from build123d import *

# Parameters (mm, degrees)
F2_DEPTH      = 24.25
F2_DEPTH_BACK = 24.25
F3_R          = 11.025
F3_R_2        = 1.75
F4_DEPTH      = 4.75
F6_DEPTH      = 15
F6_DEPTH_BACK = 15


with BuildPart() as f2:
    # F1 (on Front) → F2 (new body, two sides)
    with BuildSketch(Plane.XZ) as f2_sk:
        with BuildLine():
            ThreePointArc((-31.323529, -7.382294), (-30, 7.5), (-28.676471, -7.382294))
            ThreePointArc((-28.676471, -7.382294), (-29.266965, -7.724911), (-29.5, -8.3666))
            Line((-29.5, -8.3666), (-29.5, -11.401754))
            ThreePointArc((-29.5, -11.401754), (-29.15938, -12.153564), (-28.369565, -12.393211))
            ThreePointArc((-28.369565, -12.393211), (-19.18639, -6.270235), (-18.434131, 4.741379))
            ThreePointArc((-18.434131, 4.741379), (-18.244502, 6.614172), (-16.583592, 7.5))
            Line((-16.583592, 7.5), (16.583592, 7.5))
            ThreePointArc((16.583592, 7.5), (18.244502, 6.614172), (18.434131, 4.741379))
            ThreePointArc((18.434131, 4.741379), (19.18639, -6.270235), (28.369565, -12.393211))
            ThreePointArc((28.369565, -12.393211), (29.15938, -12.153564), (29.5, -11.401754))
            Line((29.5, -11.401754), (29.5, -8.3666))
            ThreePointArc((29.5, -8.3666), (29.266965, -7.724911), (28.676471, -7.382294))
            ThreePointArc((28.676471, -7.382294), (30, 7.5), (31.323529, -7.382294))
            ThreePointArc((31.323529, -7.382294), (30.733035, -7.724911), (30.5, -8.3666))
            Line((30.5, -8.3666), (30.5, -11.401754))
            ThreePointArc((30.5, -11.401754), (30.84062, -12.153564), (31.630435, -12.393211))
            ThreePointArc((31.630435, -12.393211), (40.81361, -6.270235), (41.565869, 4.741379))
            ThreePointArc((41.565869, 4.741379), (41.755498, 6.614172), (43.416408, 7.5))
            Line((43.416408, 7.5), (50, 7.5))
            Line((50, 7.5), (50, 12.5))
            Line((50, 12.5), (24.75, 12.5))
            Line((24.75, 12.5), (24.75, 82.5))
            Line((24.75, 82.5), (20, 82.5))
            Line((20, 82.5), (20, 12.5))
            Line((20, 12.5), (-43.416408, 12.5))
            Line((-43.416408, 12.5), (-43.416408, 7.5))
            ThreePointArc((-43.416408, 7.5), (-41.755498, 6.614172), (-41.565869, 4.741379))
            ThreePointArc((-41.565869, 4.741379), (-40.81361, -6.270235), (-31.630435, -12.393211))
            ThreePointArc((-31.630435, -12.393211), (-30.84062, -12.153564), (-30.5, -11.401754))
            Line((-30.5, -11.401754), (-30.5, -8.3666))
            ThreePointArc((-30.5, -8.3666), (-30.733035, -7.724911), (-31.323529, -7.382294))
        make_face()
    extrude(amount=F2_DEPTH)
    extrude(f2_sk.sketch, amount=-F2_DEPTH_BACK)

    # F3 (on face) → F4 (cut, through all)
    with BuildSketch(Plane(origin=(20, 0, 0), x_dir=(0, -1, 0), z_dir=(-1, 0, 0))):
        with Locations((1.9, 58.65)):
            Circle(F3_R)
        with Locations((-13.6, 43.15)):
            Circle(F3_R_2)
        with Locations((17.4, 43.15)):
            Circle(F3_R_2)
        with Locations((17.4, 74.15)):
            Circle(F3_R_2)
        with Locations((-13.6, 74.15)):
            Circle(F3_R_2)
    extrude(amount=-F4_DEPTH, mode=Mode.SUBTRACT)

    # F5 (on Front) → F6 (join, two sides)
    with BuildSketch(Plane.XZ) as f6_sk:
        Polygon((-10, -11.5), (-10, 9.493519), (-19.701663, 9.493519), (-19.701663, 0), (-27.352255, -11.5), align=None)
    extrude(amount=F6_DEPTH)
    extrude(f6_sk.sketch, amount=-F6_DEPTH_BACK)


solid = f2.part
Here's how the part is built. I have some questions about the finished solid (model axes, mm). A direction names the side the tool comes from. Give positions to 0.01 mm unless a question says otherwise; leave off trailing zeros. Loops run counter-clockwise (first coordinate to the right, second up) from the corner with the lowest first, then second, coordinate; pieces in that order, holes last. Notation, with made-up numbers: (-40, 29.25) -> (18, 29.25) arc R27 cw to (18, 53.25) -> close; hole circle Ø3 at (54.5, -19). An arc over 180 degrees is marked (long way). Answer as a JSON object with one key per item and string values. Group by question number.
Item 1: On a 3-axis mill with a long thin cutter (end or side, diameter ignored), from which of +Z, -Z, +X, -X, +Y, -Y can I reach the whole of each face in a straight line? I mean faces 1 (the cylindrical face through (-18.26, 19.56, 6.59)), 2 (the flat face through (24.75, 0, 47)), 3 (the flat face through (-29.5, 0, -10)). Say none if no direction works.
Item 2: Thinking about a two-plate mould opening in Z: for faces 4 (the cylindrical face through (-41.771, -0.34, 6.637)), 5 (the cylindrical face through (40.73, -0.34, -6.41)), 6 (the flat face through (-18, 0, -11.5)), 7 (the flat face through (-10, 0, -2)), which applies, pulls with the +Z half, pulls with the -Z half, needs draft (parallel to the pull), parting line crosses it, or undercut?
Item 3: I need wall thicknesses on L1, parallel to Y at x = 22.85, z = 74.15; L2, parallel to X at y = 0, z = 0; L3, parallel to X at y = 19, z = 2. Which ranges of each line are inside material? Lowest first, please.
Item 4: Will these pins go through, and if not, where does the flat tip stop? pin 1 (0.9 mm diameter, centred on y = 2, z = -9.5, fed in from -X); pin 2 (12 mm diameter, centred on y = 3.5, z = 52.5, fed in from +X); pin 3 (8 mm diameter, centred on x = 37, y = 2, fed in from -Z).
Item 5: Imagine slicing it at C-C on z = -0.5. Write out the boundary of the cut face in (x, y), then the cut area to 3 significant figures.
Item 6: Imagine slicing it at A-A on z = 43.15. Write out the boundary of the cut face in (x, y), then the cut area to 3 significant figures.
Item 7: Imagine slicing it at B-B on x = 33. Write out the boundary of the cut face in (y, z).
Answer list:
{
 "1": {"face 1": "+Y", "face 2": "+Z, +X, +Y, -Y", "face 3": "-Z, +Y, -Y"},
 "2": {"face 4": "undercut", "face 5": "undercut", "face 6": "pulls with the -Z half", "face 7": "needs draft"},
 "3": {"L1": "y = -24.25 to -19.15, -15.65 to 11.85, 15.35 to 24.25", "L2": "x = -42.5 to -37.5, -22.5 to -10, 17.5 to 22.5, 37.5 to 42.5", "L3": "x = -42.34 to -37.23, -22.77 to -17.66, 17.66 to 22.77, 37.23 to 42.34"},
 "4": {"pin 1": "stops at x = -38.62", "pin 2": "stops at x = 24.75", "pin 3": "stops at z = -12.13"},
 "5": {"outline": "(-42.49, -24.25) -> (-37.48, -24.25) -> (-37.48, 24.25) -> (-42.49, 24.25) -> close; (-22.52, -24.25) -> (-17.51, -24.25) -> (-17.51, -15) -> (-10, -15) -> (-10, 15) -> (-17.51, 15) -> (-17.51, 24.25) -> (-22.52, 24.25) -> close; (17.51, -24.25) -> (22.52, -24.25) -> (22.52, 24.25) -> (17.51, 24.25) -> close; (37.48, -24.25) -> (42.49, -24.25) -> (42.49, 24.25) -> (37.48, 24.25) -> close", "area": "1,200 mm2"},
 "6": {"outline": "(20, -24.25) -> (24.75, -24.25) -> (24.75, -19.15) -> (20, -19.15) -> close; (20, -15.65) -> (24.75, -15.65) -> (24.75, 11.85) -> (20, 11.85) -> close; (20, 15.35) -> (24.75, 15.35) -> (24.75, 24.25) -> (20, 24.25) -> close", "area": "197 mm2"},
 "7": {"outline": "(-24.25, -12.13) -> (24.25, -12.13) -> (24.25, -6.87) -> (-24.25, -6.87) -> close; (-24.25, 6.87) -> (24.25, 6.87) -> (24.25, 12.5) -> (-24.25, 12.5) -> close"}
}
